```python
from build123d import *

# Parameters (mm, degrees)
BASE_FLANGE1_DEPTH             = 2.286
EDGE_FLANGE1_STRIP_W           = 11.43
EDGE_FLANGE1_STRIP_H           = 2.286
EDGE_FLANGE1_STRIP_CUT_DEPTH   = 71.239731207
EDGE_FLANGE1_STRIP_2_W         = 11.43
EDGE_FLANGE1_STRIP_2_H         = 2.286
EDGE_FLANGE1_STRIP_CUT_2_DEPTH = 50.8
EDGE_FLANGE1_STRIP_3_W         = 11.43
EDGE_FLANGE1_STRIP_3_H         = 2.286
EDGE_FLANGE1_STRIP_CUT_3_DEPTH = 84.622425054
EDGE_FLANGE1_DEPTH             = 71.239731207
EDGE_FLANGE1_BEND_DEPTH        = 50.8
EDGE_FLANGE1_BEND_2_DEPTH      = 84.622425054


# Sheet-metal steps are written as plain solids
with BuildPart() as part:
    # Sketch1 → Base-Flange1 (new body)
    with BuildSketch(Plane.XY):
        Polygon((0, 0), (0, -6.35), (50.8, -6.35), (50.8, 0), (56.291897179, 3.187721032), (13.811159523, 76.374753696), (4.964395568, 71.239731207), (-6.35, 71.239731207), (-6.35, 0), align=None)
    extrude(amount=-BASE_FLANGE1_DEPTH)

    # Edge-Flange1 strip (across the edge) → Edge-Flange1 strip cut (cut)
    with BuildSketch(Plane(origin=(-6.35, 71.239731207, 0), x_dir=(1, 0, 0), z_dir=(0, -1, 0))):
        with Locations((-2.286, -1.143)):
            Rectangle(EDGE_FLANGE1_STRIP_W, EDGE_FLANGE1_STRIP_H)
    extrude(amount=EDGE_FLANGE1_STRIP_CUT_DEPTH, mode=Mode.SUBTRACT)

    # Edge-Flange1 strip 2 (across the edge) → Edge-Flange1 strip cut 2 (cut)
    with BuildSketch(Plane(origin=(0, -6.35, 0), x_dir=(0, 1, 0), z_dir=(1, 0, 0))):
        with Locations((-2.286, -1.143)):
            Rectangle(EDGE_FLANGE1_STRIP_2_W, EDGE_FLANGE1_STRIP_2_H)
    extrude(amount=EDGE_FLANGE1_STRIP_CUT_2_DEPTH, mode=Mode.SUBTRACT)

    # Edge-Flange1 strip 3 (across the edge) → Edge-Flange1 strip cut 3 (cut)
    with BuildSketch(Plane(origin=(56.291897179, 3.187721032, 0), x_dir=(-0.8648656974537777, -0.5020033121083872, 3.491481338843133e-15), z_dir=(-0.5020033121083872, 0.8648656974537777, 0))):
        with Locations((-2.286, -1.143)):
            Rectangle(EDGE_FLANGE1_STRIP_3_W, EDGE_FLANGE1_STRIP_3_H)
    extrude(amount=EDGE_FLANGE1_STRIP_CUT_3_DEPTH, mode=Mode.SUBTRACT)

    # Edge-Flange1 section (across the edge) → Edge-Flange1 (add)
    with BuildSketch(Plane(origin=(-6.35, 71.239731207, 0), x_dir=(1, 0, 0), z_dir=(0, -1, 0))):
        with BuildLine():
            Line((0, 1.143), (0, 10.414))
            Line((0, 10.414), (2.286, 10.414))
            Line((2.286, 10.414), (2.286, 1.143))
            ThreePointArc((2.286, 1.143), (2.620776949, 0.334776949), (3.429, 0))
            Line((3.429, 0), (3.429, -2.286))
            ThreePointArc((3.429, -2.286), (1.004330847, -1.281669153), (0, 1.143))
        make_face()
    extrude(amount=EDGE_FLANGE1_DEPTH)

    # Edge-Flange1 section 2 (across the edge) → Edge-Flange1 bend (add)
    with BuildSketch(Plane(origin=(0, -6.35, 0), x_dir=(0, 1, 0), z_dir=(1, 0, 0))):
        with BuildLine():
            Line((0, 1.143), (0, 10.414))
            Line((0, 10.414), (2.286, 10.414))
            Line((2.286, 10.414), (2.286, 1.143))
            ThreePointArc((2.286, 1.143), (2.620776949, 0.334776949), (3.429, 0))
            Line((3.429, 0), (3.429, -2.286))
            ThreePointArc((3.429, -2.286), (1.004330847, -1.281669153), (0, 1.143))
        make_face()
    extrude(amount=EDGE_FLANGE1_BEND_DEPTH)

    # Edge-Flange1 section 3 (across the edge) → Edge-Flange1 bend 2 (add)
    with BuildSketch(Plane(origin=(56.291897179, 3.187721032, 0), x_dir=(-0.8648656974537777, -0.5020033121083872, 3.491481338843133e-15), z_dir=(-0.5020033121083872, 0.8648656974537777, 0))):
        with BuildLine():
            Line((0, 1.143), (0, 10.414))
            Line((0, 10.414), (2.286, 10.414))
            Line((2.286, 10.414), (2.286, 1.143))
            ThreePointArc((2.286, 1.143), (2.620776949, 0.334776949), (3.429, 0))
            Line((3.429, 0), (3.429, -2.286))
            ThreePointArc((3.429, -2.286), (1.004330847, -1.281669153), (0, 1.143))
        make_face()
    extrude(amount=EDGE_FLANGE1_BEND_2_DEPTH)


solid = part.part
```
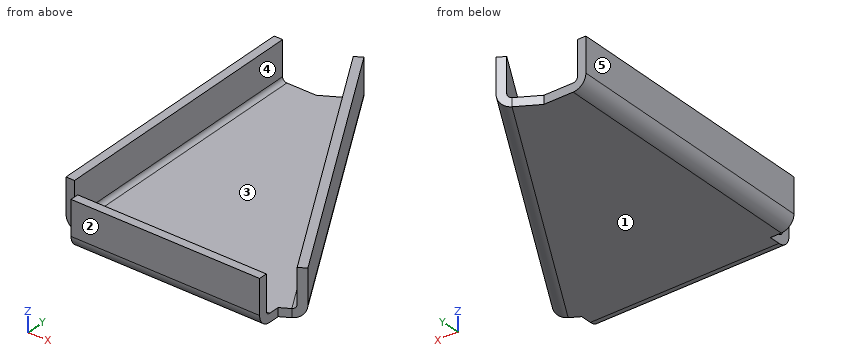
Work out the finished part from the listing and answer in its coordinate system (mm). Face numbers are marked on the shaded views. A direction names the side the tool comes from. Coordinates: 2 decimals unless noted, no trailing zeros. Write each loop counter-clockwise with the first axis right and the second up, starting at its lowest first coordinate (ties: lowest second). Pieces come first, ordered by that corner, then holes.
Q1. A cutting plane is placed at A-A, the plane z = 3. Give the vertices of the cut face in (x, y), then the cut area to 3 significant figures.
Q2. Find the intervals of material crossed by line 1 (Z direction, x = 49.5, y = 2); line 2 (X direction, y = 5, z = 7.25); line 3 (X direction, y = 63, z = 4), in increasing order.
Q3. Which of the six approach directions +Z, -Z, +X, -X, +Y, -Y give full straight-line access (tool end or side, diameter ignored) to the marked faces 4 and 5?
Q4. Each of these flat-tipped pins is pushed along its axis until it touches: pin 1 Ø1.5 at (y, z) = (65, 7) entering from +X; pin 2 Ø7 at (y, z) = (-3, 4) entering from +X; pin 3 Ø5 at (x, y) = (47, 10.5) entering from +Z; pin 4 Ø4 at (y, z) = (26.5, 0) entering from +X. Where does it stop, or does it pass through?
Q5. A cutting plane is placed at C-C, the plane y = -1. Give the vertices of the cut face in (x, z).
Q6. Determine the mould class of the marked faces 1, 2 and 3 for opening direction Y: released by +Y, released by -Y, zero draft, split by the parting line, or undercut.
Q7. A cutting plane is placed at B-B, the plane x = 6. Give the vertices of the cut face in (y, z), then the cut area to 3 significant figures.
Findings below:
1. outline: (-6.35, 0) - (-4.06, 0) - (-4.06, 71.24) - (-6.35, 71.24) - close; (0, -6.35) - (50.8, -6.35) - (50.8, -4.06) - (0, -4.06) - close; (11.83, 75.23) - (54.31, 2.04) - (56.29, 3.19) - (13.81, 76.37) - close
1. area: 472 mm2
2. line 1: z = -2.29 to 0
2. line 2: x = -6.35 to -4.06, 52.6 to 55.24
2. line 3: x = -6.35 to -4.06, 18.93 to 21.57
3. face 4: +Z, +Y, -Y
3. face 5: +Z, -Z, -X, +Y, -Y
4. pin 1: stops at x = 20.85
4. pin 2: stops at x = 50.8
4. pin 3: stops at z = 10.41
4. pin 4: stops at x = 43.82
5. outline: (0, -2.29) - (50.8, -2.29) - (50.8, 0) - (0, 0) - close
6. face 1: zero draft
6. face 2: released by -Y
6. face 3: undercut
7. outline: (-6.35, 1.14) arc R3.43 ccw to (-2.92, -2.29) - (71.84, -2.29) - (71.84, 0) - (-2.92, 0) arc R1.14 cw to (-4.06, 1.14) - (-4.06, 10.41) - (-6.35, 10.41) - close
7. area: 200 mm2
